```python
from build123d import *

# Parameters (mm, degrees)
BOSS_EXTRUDE1_DEPTH = 3
FILLET1_R           = 4
BOSS_EXTRUDE2_DEPTH = 1
CUT_EXTRUDE1_REACH  = 72.897
SKETCH5_R           = 1.55


with BuildPart() as part:
    # Sketch1 → Boss-Extrude1 (new body)
    with BuildSketch(Plane.XY):
        Polygon((49.961918802, 33.053079846), (25.841829778, 39.627371101), (24.789943177, 35.768156857), (24.184782156, 33.547911794), (33.022732651, 24.493907566), (48.796245804, 28.776400372), align=None)
        Polygon((27.4988774, 45.706830407), (26.893716379, 43.486585345), (25.841829778, 39.627371101), (49.961918802, 33.053079846), (51.127591799, 37.329759319), (39.708758261, 49.023933188), align=None)
        with BuildLine():
            Line((24.964109257, 44.012528645), (5.668038039, 49.271961649))
            Line((5.668038039, 49.271961649), (4.616151438, 45.412747405))
            ThreePointArc((4.616151438, 45.412747405), (5.002692971, 42.375780391), (7.423479081, 40.501646561))
            Line((7.423479081, 40.501646561), (24.789943177, 35.768156857))
            Line((24.789943177, 35.768156857), (25.841829778, 39.627371101))
            Line((25.841829778, 39.627371101), (26.893716379, 43.486585345))
            Line((26.893716379, 43.486585345), (24.964109257, 44.012528645))
        make_face()
    extrude(amount=BOSS_EXTRUDE1_DEPTH)

    # Fillet1
    fillet1_edges = [part.edges().sort_by_distance(p)[0] for p in [
        (5.668038039, 49.271961649, 1.5),
    ]]
    fillet(fillet1_edges, radius=FILLET1_R - 0.0001)  # a hair under: the kernel refuses the full size

    # Sketch2 → Boss-Extrude2 (add)
    with BuildSketch(Plane.XY.offset(3)):
        Polygon((48.796245804, 28.776400372), (33.022732651, 24.493907566), (24.184782156, 33.547911794), (24.789943177, 35.768156857), (26.893716379, 43.486585345), (27.4988774, 45.706830407), (39.708758261, 49.023933188), (51.127591799, 37.329759319), align=None)
        Polygon((27.85851994, 43.223613694), (25.754746738, 35.505185207), (25.300052744, 33.836981106), (33.327840747, 25.612944712), (47.98193766, 29.591517145), (50.012292821, 37.040585847), (39.40383219, 47.904846429), (28.313213935, 44.891817795), align=None, mode=Mode.SUBTRACT)
    extrude(amount=BOSS_EXTRUDE2_DEPTH)

    # Sketch5 → Cut-Extrude1 (cut, up to next)
    with BuildSketch(Plane.XY.offset(3), mode=Mode.PRIVATE) as cut_extrude1_sk1:
        with Locations((8.475365681, 44.360860805)):
            Circle(SKETCH5_R)
    cut_extrude1_tool1 = extrude(cut_extrude1_sk1.sketch, amount=-CUT_EXTRUDE1_REACH, mode=Mode.PRIVATE) & part.part
    # Sketch5 → Cut-Extrude1 (cut, up to next)
    with BuildSketch(Plane.XY.offset(3), mode=Mode.PRIVATE) as cut_extrude1_sk2:
        with Locations((20.053008413, 41.205201002)):
            Circle(SKETCH5_R)
    cut_extrude1_tool2 = extrude(cut_extrude1_sk2.sketch, amount=-CUT_EXTRUDE1_REACH, mode=Mode.PRIVATE) & part.part
    add(cut_extrude1_tool1.solids().sort_by_distance((8.475366, 44.360861, 3))[0], mode=Mode.SUBTRACT)
    add(cut_extrude1_tool2.solids().sort_by_distance((20.053008, 41.205201, 3))[0], mode=Mode.SUBTRACT)


solid = part.part
```
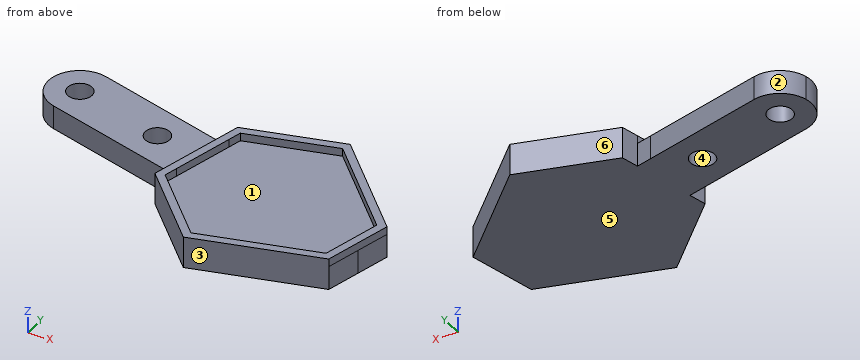
Model file for the job. Use its own axes, mm. Face numbers are marked on the shaded views. A direction names the side the tool comes from. Round coordinates to 2 decimals unless told otherwise and drop trailing zeros. Order: outer loops, then holes, each group sorted by start corner. A loop starts at its lowest first (then second) coordinate and runs counter-clockwise, first axis right, second up. Notation, with made-up numbers: (51, -38) -> (106, -38) arc R25 ccw to (106, -13) -> close; hole circle Ø1 at (85.5, 79). An arc over 180 degrees is marked (long way). Use one line per item in the form item = value.
Item 1: Cut at B-B, the plane z = 3.45. Write the cut outline in (x, y).
Returned:
outline = (24.18, 33.55) -> (33.02, 24.49) -> (48.8, 28.78) -> (51.13, 37.33) -> (39.71, 49.02) -> (27.5, 45.71) -> close; hole (25.3, 33.84) -> (33.33, 25.61) -> (47.98, 29.59) -> (50.01, 37.04) -> (39.4, 47.9) -> (28.31, 44.89) -> close
Item 2: Cut at D-D, the plane x = 36. Write the cut outline in (y, z).
Returned:
outline = (25.3, 0) -> (48.02, 0) -> (48.02, 4) -> (46.98, 4) -> (46.98, 3) -> (26.34, 3) -> (26.34, 4) -> (25.3, 4) -> close
Item 3: Flat gauge pins, fed straight in: pin 1 Ø1.9 at (x, y) = (20.05, 41.21) entering from -Z; pin 2 Ø1.5 at (y, z) = (27.5, 0.5) entering from -X; pin 3 Ø1.5 at (x, y) = (14, 45.5) entering from +Z. Where does each tip first touch, or does it go through?
Returned:
pin_1 = through
pin_2 = 29.36
pin_3 = 3
Item 4: Cut at A-A, the plane y = 41.75. Write the cut outline in (x, z).
Returned:
outline = (5.44, 0) -> (18.6, 0) -> (18.6, 3) -> (5.44, 3) -> close; (21.5, 0) -> (46.81, 0) -> (46.81, 4) -> (45.41, 4) -> (45.41, 3) -> (27.46, 3) -> (27.46, 4) -> (26.42, 4) -> (26.42, 3) -> (21.5, 3) -> close
Item 5: Pull direction Y, two halves, no side cores. Call the marked faces 1, 2, 3 and 4: released by +Y, released by -Y, zero draft, split by the parting line, or undercut.
Returned:
face_1 = undercut
face_2 = released by +Y
face_3 = released by -Y
face_4 = undercut
Item 6: Cut at C-C, the plane z = 0.5. Give the number of separate pieces and of enclosed holes in the cut face, and give its area (3 significant figures).
Returned:
separate_pieces = 1
enclosed_holes = 2
area = 603 mm^2
Item 7: Drill centre lines: line 1 (Z direction, x = 12.5, y = 45); line 2 (X direction, y = 43, z = 0.55); line 3 (Y direction, x = 20, z = 1.4). Where is each one in solid material? Low to high.
Returned:
line_1 = 0 to 3
line_2 = 4.71 to 7.73, 9.22 to 45.59
line_3 = 37.07 to 39.66, 42.75 to 45.37
Item 8: Tool access for the marked faces 5 and 6: list every direction of +Z, -Z, +X, -X, +Y, -Y with a clear straight run to the whole face (end or side of a thin tool).
Returned:
face_5 = -Z, +X, -X, +Y, -Y
face_6 = +Z, -Z, +Y
